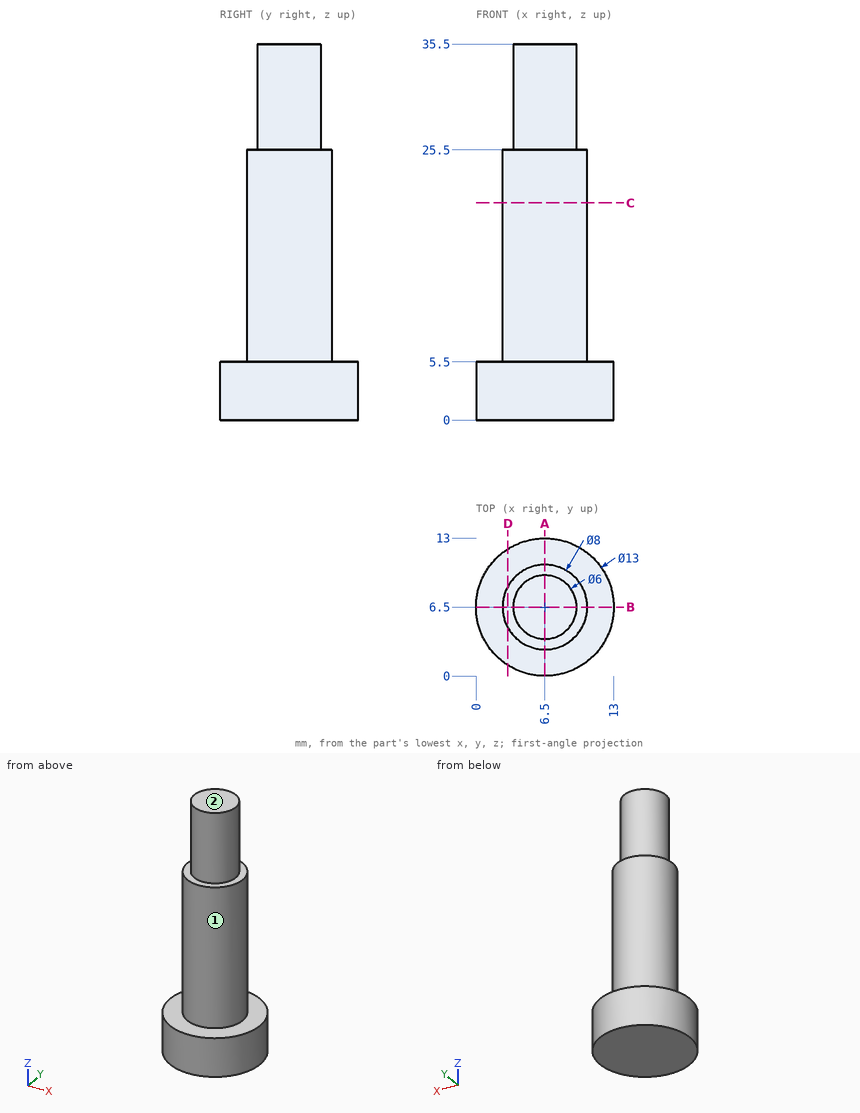
Design review of the part shown in the three views and the two pictorial views. Dimensions are in mm from the part's minimum x, y and z. A direction names the side the tool comes from. Round coordinates to 2 decimals unless told otherwise and drop trailing zeros. Order: outer loops, then holes, each group sorted by start corner. A loop starts at its lowest first (then second) coordinate and runs counter-clockwise, first axis right, second up.
Item 1: Machinability: for the marked faces 1 and 2, which of the approach directions +Z, -Z, +X, -X, +Y, -Y give a long, thin tool a straight path to every point of the face, cutting with its end or side? Answer none if there is none.
Working result:
face 1: +Z
face 2: +Z, +X, -X, +Y, -Y
Item 2: For pin 1 (2 mm diameter, centred on x = 10, y = 3.5, fed in from +Z); pin 2 (3 mm diameter, centred on x = 5.5, z = 16.5, fed in from +Y); pin 3 (4 mm diameter, centred on x = 6, z = 20.5, fed in from -Y); pin 4 (1.5 mm diameter, centred on y = 2.5, z = 29, fed in from +X), all flat-tipped, find the tip position at first contact; note any pin that passes through.
Working result:
pin 1: stops at z = 25.5
pin 2: stops at y = 10.5
pin 3: stops at y = 2.5
pin 4: passes through
Item 3: Add section A-A, the plane x = 6.5. State the section outline as (y, z) points, and give its area (4 significant figures).
Working result:
outline: (0, 0) - (13, 0) - (13, 5.5) - (10.5, 5.5) - (10.5, 25.5) - (9.5, 25.5) - (9.5, 35.5) - (3.5, 35.5) - (3.5, 25.5) - (2.5, 25.5) - (2.5, 5.5) - (0, 5.5) - close
area: 291.5 mm2
Item 4: To check wall thickness, follow probe 1 along Z at (x, y) = (8.25, 0.75); probe 2 along X at (y, z) = (10, 19.5); probe 3 along Z at (x, y) = (3.5, 8). State the ranges of each line that lie inside material, in increasing order.
Working result:
probe 1: z = 0 to 5.5
probe 2: x = 4.56 to 8.44
probe 3: z = 0 to 25.5
Item 5: Add section D-D, the plane x = 3. State the section outline as (y, z) points, and give its area (3 significant figures).
Working result:
outline: (1.02, 0) - (11.98, 0) - (11.98, 5.5) - (8.44, 5.5) - (8.44, 25.5) - (4.56, 25.5) - (4.56, 5.5) - (1.02, 5.5) - close
area: 138 mm2
Item 6: Add section C-C, the plane z = 20.5. State the section outline as (x, y) points.
Working result:
outline: circle Ø8 at (6.5, 6.5)
